from build123d import *

# Parameters (mm, degrees)
SKETCH1_R           = 18.25
SKETCH1_R_2         = 1.6
SKETCH1_R_3         = 11.5
BOSS_EXTRUDE1_DEPTH = 2
SKETCH1_3_R         = 21.25
SKETCH1_3_R_2       = 18.25
BOSS_EXTRUDE2_DEPTH = 32
BOSS_EXTRUDE3_DEPTH = 32


with BuildPart() as part:
    # Sketch1 → Boss-Extrude1 (new body)
    with BuildSketch(Plane(origin=(0, 0, 0), x_dir=(1, 0, 0), z_dir=(0, 1, 0))):
        with Locations(Location((0, 0, 0), (0, 0, 270))):
            Circle(SKETCH1_R)
        with Locations(Location((-14, 0, 0), (0, 0, 270))):
            Circle(SKETCH1_R_2, mode=Mode.SUBTRACT)
        with Locations(Location((0, -14, 0), (0, 0, 270))):
            Circle(SKETCH1_R_2, mode=Mode.SUBTRACT)
        with Locations(Location((14, 0, 0), (0, 0, 270))):
            Circle(SKETCH1_R_2, mode=Mode.SUBTRACT)
        with Locations(Location((0, 14, 0), (0, 0, 270))):
            Circle(SKETCH1_R_2, mode=Mode.SUBTRACT)
        with Locations(Location((0, 0, 0), (0, 0, 270))):
            Circle(SKETCH1_R_3, mode=Mode.SUBTRACT)
    extrude(amount=BOSS_EXTRUDE1_DEPTH)

    # Sketch1_3 → Boss-Extrude2 (add)
    with BuildSketch(Plane(origin=(0, 0, 0), x_dir=(1, 0, 0), z_dir=(0, 1, 0))):
        with Locations(Location((0, 0, 0), (0, 0, 270))):
            Circle(SKETCH1_3_R)
        with Locations(Location((0, 0, 0), (0, 0, 270))):
            Circle(SKETCH1_3_R_2, mode=Mode.SUBTRACT)
    extrude(amount=BOSS_EXTRUDE2_DEPTH)

    # Sketch2 → Boss-Extrude3 (add)
    with BuildSketch(Plane(origin=(0, 0, 0), x_dir=(1, 0, 0), z_dir=(0, 1, 0))):
        with BuildLine():
            ThreePointArc((5.4e-08, -21.25), (-15.026019081, -15.026019119), (-21.25, 0))
            Line((-21.25, 0), (-21.25, -21.25))
            Line((-21.25, -21.25), (5.4e-08, -21.25))
        make_face()
        with BuildLine():
            Line((21.25, -21.25), (21.25, 0))
            ThreePointArc((21.25, 0), (15.026019119, -15.026019081), (5.4e-08, -21.25))
            Line((5.4e-08, -21.25), (21.25, -21.25))
        make_face()
    extrude(amount=BOSS_EXTRUDE3_DEPTH)


solid = part.part
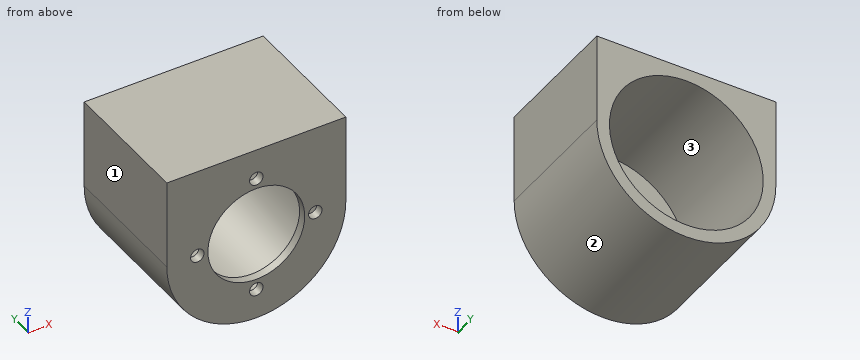
Design review of the part built by this model. Coordinates are the model's own, in mm. Face numbers are marked on the shaded views. Coordinates: 2 decimals unless noted, no trailing zeros. Order: outer loops, then holes, each group sorted by start corner. A loop starts at its lowest first (then second) coordinate and runs counter-clockwise, first axis right, second up. Notation, with made-up numbers: (89.25, 12.5) - (115.25, 12.5) arc R7 ccw to (115.25, 20.5) - close; hole circle Ø9 at (15.5, 9.25). An arc over 180 degrees is marked (long way). Put each result on its own line as item: value.
1) Take a section at D-D, the plane x = -8. Give the boundary of the cut face in (y, z).
Response values:
outline: (0, -19.69) - (32, -19.69) - (32, -16.4) - (2, -16.4) - (2, -8.26) - (0, -8.26) - close; (0, 8.26) - (2, 8.26) - (2, 16.4) - (32, 16.4) - (32, 21.25) - (0, 21.25) - close
2) Insertion check: P1, Ø2, axis at x = -10, z = -8, coming from the +Y side; P2, Ø18.5, axis at x = 0, z = 0, coming from the -Y side; P3, Ø10, axis at y = 27, z = -15, coming from the -X side; P4, Ø5, axis at y = 28, z = -4.5, coming from the -X side. Each pin has a flat end and moves straight along its axis. Give the tip position at first contact, or say it passes through.
Response values:
P1: stops at y = 2
P2: passes through
P3: stops at x = -18.75
P4: stops at x = -21.16
3) The part is to be moulded in two halves that separate along Z. For the marked faces 1, 2 and 3, say which applies: released by +Z, released by -Z, zero draft, split by the parting line, or undercut.
Response values:
face 1: zero draft
face 2: released by -Z
face 3: undercut
4) Take a section at B-B, the plane x = 0. Give the boundary of the cut face in (y, z).
Response values:
outline: (0, -21.25) - (32, -21.25) - (32, -18.25) - (2, -18.25) - (2, -15.6) - (0, -15.6) - close; (0, -12.4) - (2, -12.4) - (2, -11.5) - (0, -11.5) - close; (0, 11.5) - (2, 11.5) - (2, 12.4) - (0, 12.4) - close; (0, 15.6) - (2, 15.6) - (2, 18.25) - (32, 18.25) - (32, 21.25) - (0, 21.25) - close
5) Wall thickness on L1, parallel to X at y = 0.7, z = 0; L2, parallel to X at y = 1.25, z = 14; L3, parallel to Z at x = -9, y = 4: over which ranges is each line inside the solid? List them lowest first. Write a range as from..to.
Response values:
L1: x = -21.25..-15.6, -12.4..-11.5, 11.5..12.4, 15.6..21.25
L2: x = -21.25..-1.6, 1.6..21.25
L3: z = -19.25..-15.88, 15.88..21.25
6) Take a section at C-C, the plane y = 14. Give the boundary of the cut face in (x, z).
Response values:
outline: (-21.25, 0) arc R21.25 ccw to (21.25, 0) - (21.25, 21.25) - (-21.25, 21.25) - close; hole circle Ø36.5 at (0, 0)
7) Take a section at A-A, the plane z = 2.5. Give the boundary of the cut face in (x, y), and give its area (3 significant figures).
Response values:
outline: (-21.25, 0) - (-11.22, 0) - (-11.22, 2) - (-18.08, 2) - (-18.08, 32) - (-21.25, 32) - close; (11.22, 0) - (21.25, 0) - (21.25, 32) - (18.08, 32) - (18.08, 2) - (11.22, 2) - close
area: 230 mm²
